```python
from build123d import *

# Parameters (mm, degrees)
DODANIE_WYCI_GNI_CIE1_DEPTH      = 13.5
DODANIE_WYCI_GNI_CIE1_DEPTH_BACK = 13.5
SZKIC1_W                         = 40
SZKIC1_H                         = 35
SZKIC1_R                         = 2.5
SZKIC2_R                         = 6
DODANIE_WYCI_GNI_CIE2_DEPTH      = 15
SZKIC2_4_R                       = 3
WYTNIJ_WYCI_GNI_CIE2_DEPTH       = 40
DODANIE_WYCI_GNI_CIE3_START      = -55
SZKIC2_6_R                       = 6
DODANIE_WYCI_GNI_CIE3_DEPTH      = 15
DODANIE_WYCI_GNI_CIE4_START      = 35
SZKIC3_R                         = 12
SZKIC3_W                         = 9
SZKIC3_H                         = 9
DODANIE_WYCI_GNI_CIE4_DEPTH      = 3
DODANIE_WYCI_GNI_CIE5_START      = 35
SZKIC3_3_W                       = 9
SZKIC3_3_H                       = 9
SZKIC3_3_R                       = 2
DODANIE_WYCI_GNI_CIE5_DEPTH      = 10


with BuildPart() as part:
    # Szkic1 → Dodanie-wyci_gni_cie1 (new, two sides: drawn at the far end of the back side and taken through both)
    with BuildSketch(Plane.XY.offset(-DODANIE_WYCI_GNI_CIE1_DEPTH_BACK)):
        with Locations((20, 17.5)):
            Rectangle(SZKIC1_W, SZKIC1_H)
        with Locations((5.5, 30.5)):
            Circle(SZKIC1_R, mode=Mode.SUBTRACT)
        with Locations((34.5, 30.5)):
            Circle(SZKIC1_R, mode=Mode.SUBTRACT)
    extrude(amount=DODANIE_WYCI_GNI_CIE1_DEPTH + DODANIE_WYCI_GNI_CIE1_DEPTH_BACK)

    # Szkic2 → Dodanie-wyci_gni_cie2 (add)
    with BuildSketch(Plane(origin=(40, 0, 0), x_dir=(0, 0, -1), z_dir=(1, 0, 0))):
        Polygon((-12.701705922, 14), (-6.350852961, 3), (6.350852961, 3), (12.701705922, 14), (6.350852961, 25), (-6.350852961, 25), align=None)
        with Locations((0, 14)):
            Circle(SZKIC2_R, mode=Mode.SUBTRACT)
    extrude(amount=DODANIE_WYCI_GNI_CIE2_DEPTH)

    # Szkic2_4 → Wytnij-wyci_gni_cie2 (cut)
    with BuildSketch(Plane(origin=(40, 0, 0), x_dir=(0, 0, -1), z_dir=(1, 0, 0))):
        with Locations((0, 14)):
            Circle(SZKIC2_4_R)
    extrude(amount=-WYTNIJ_WYCI_GNI_CIE2_DEPTH, mode=Mode.SUBTRACT)

    # Szkic2_6 → Dodanie-wyci_gni_cie3 (add)
    with BuildSketch(Plane(origin=(40, 0, 0), x_dir=(0, 0, -1), z_dir=(1, 0, 0)).offset(DODANIE_WYCI_GNI_CIE3_START)):
        Polygon((-12.701705922, 14), (-6.350852961, 3), (6.350852961, 3), (12.701705922, 14), (6.350852961, 25), (-6.350852961, 25), align=None)
        with Locations((0, 14)):
            Circle(SZKIC2_6_R, mode=Mode.SUBTRACT)
    extrude(amount=DODANIE_WYCI_GNI_CIE3_DEPTH)

    # Szkic3 → Dodanie-wyci_gni_cie4 (add)
    with BuildSketch(Plane(origin=(0, 0, 0), x_dir=(1, 0, 0), z_dir=(0, 1, 0)).offset(DODANIE_WYCI_GNI_CIE4_START)):
        with Locations(Location((21, 0, 0), (0, 0, 90))):
            Circle(SZKIC3_R)
        with Locations((21, 0)):
            Rectangle(SZKIC3_W, SZKIC3_H, mode=Mode.SUBTRACT)
    extrude(amount=DODANIE_WYCI_GNI_CIE4_DEPTH)

    # Szkic3_3 → Dodanie-wyci_gni_cie5 (add)
    with BuildSketch(Plane(origin=(0, 0, 0), x_dir=(1, 0, 0), z_dir=(0, 1, 0)).offset(DODANIE_WYCI_GNI_CIE5_START)):
        with Locations((21, 0)):
            Rectangle(SZKIC3_3_W, SZKIC3_3_H)
        with Locations(Location((21, 0, 0), (0, 0, 270))):
            Circle(SZKIC3_3_R, mode=Mode.SUBTRACT)
    extrude(amount=DODANIE_WYCI_GNI_CIE5_DEPTH)


solid = part.part
```
Work out the finished part from the listing and answer in its coordinate system (mm). A direction names the side the tool comes from. Give positions to 0.01 mm unless a question says otherwise; leave off trailing zeros. Order: outer loops, then holes, each group sorted by start corner. A loop starts at its lowest first (then second) coordinate and runs counter-clockwise, first axis right, second up. Notation, with made-up numbers: (34, -28.5) -> (63, -28.5) arc R14 ccw to (63, -3.5) -> close; hole circle Ø8 at (-3.5, 17.5). An arc over 180 degrees is marked (long way). Answer as CSV lines item,"result". Start each with the question number.
(1) Section C-C, the plane x = 21 is taken. Write down the section's boundary in (y, z).
(2) Which of the six approach directions +Z, -Z, +X, -X, +Y, -Y give full straight-line access (tool end or side, diameter ignored) to faces 1 (the flat face through (16.5, 41, 0)), 2 (the flat face through (-8, 3, 0)), 3 (the cylindrical face through (23, 40, 0))?
(3) Each of these flat-tipped pins is pushed along its axis until it touches: pin 1 Ø1.5 at (y, z) = (10.5, -4.5) entering from -X; pin 2 Ø7 at (y, z) = (14, 0) entering from -X; pin 3 Ø3 at (x, y) = (20, 39) entering from -Z; pin 4 Ø6 at (x, y) = (44.5, 14.5) entering from +Z. Where does it stop, or does it pass through?
(4) For a pull along Z with two mould halves and no side action, classify faces 4 (the flat face through (21, 38, -5)), 5 (the flat face through (47.4, 19.58, 9.48)), 6 (the cylindrical face through (47, 14, 6)) as released by +Z, released by -Z, zero draft, split by the parting line, or undercut.
(5) Section D-D, the plane z = 0 is taken. Give the number of separate pieces and of enclosed holes in the cut face, plus the area to 3 significant figures.
(6) Consider line 1 along X through (y, z) = (29, -6.5); line 2 along Y through (x, z) = (20, 0); line 3 along X through (y, z) = (32.5, -11.5). Determine where each line is inside the solid, lowest interval first.
(7) Section A-A, the plane x = 5.5 is taken. Write down the section's boundary in (y, z), plus the area to 3 significant figures.
(8) Section B-B, the plane y = 30.5 is taken. Write down the section's boundary in (x, z).
Entries:
1,outline,"(0, -13.5) -> (35, -13.5) -> (35, -12) -> (38, -12) -> (38, -4.5) -> (45, -4.5) -> (45, -2) -> (35, -2) -> (35, 2) -> (45, 2) -> (45, 4.5) -> (38, 4.5) -> (38, 12) -> (35, 12) -> (35, 13.5) -> (0, 13.5) -> close; hole circle Ø6 at (14, 0)"
2,face 1,"+Z, -Z, -X, +Y"
2,face 2,"+Z, -Z, -X, -Y"
2,face 3,"+Y"
3,pin 1,"x = -15"
3,pin 2,"x = 0"
3,pin 3,"z = -12"
3,pin 4,"z = 12.7"
4,face 4,"zero draft"
4,face 5,"released by +Z"
4,face 6,"undercut"
5,separate pieces,"2"
5,enclosed holes,"2"
5,area,"1,520 mm²"
6,line 1,"0 to 3.5, 7.5 to 32.5, 36.5 to 40"
6,line 2,"0 to 11, 17 to 35"
6,line 3,"0 to 4, 7 to 33, 36 to 40"
7,outline,"(0, -13.5) -> (28, -13.5) -> (28, 13.5) -> (0, 13.5) -> close; (33, -13.5) -> (35, -13.5) -> (35, 13.5) -> (33, 13.5) -> close; hole circle Ø6 at (14, 0)"
7,area,"782 mm²"
8,outline,"(0, -13.5) -> (3, -13.5) -> (3, 13.5) -> (0, 13.5) -> close; (8, -13.5) -> (32, -13.5) -> (32, 13.5) -> (8, 13.5) -> close; (37, -13.5) -> (40, -13.5) -> (40, 13.5) -> (37, 13.5) -> close"
